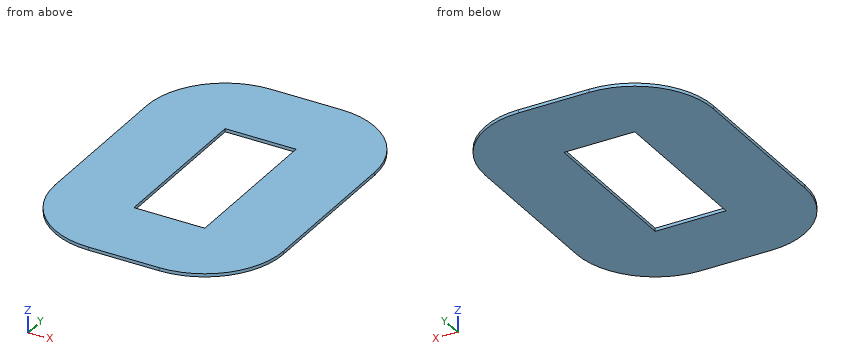
Solid Edge part; units mm, degrees
sketch "Sketch1" plane through (0, 0, 0) normal (0, 0, 1) x (1, 0, 0)
  arc A0 (-55.4402, 24.709) -> (-45.4402, 34.709) centre (-45.4402, 24.709) cw
  line L0 (-36.4402, 34.709) -> (-45.4402, 34.709)
  arc A1 (-36.4402, 34.709) -> (-26.4402, 24.709) centre (-36.4402, 24.709) cw
  line L1 (-26.4402, 4.709) -> (-26.4402, 24.709)
  arc A2 (-26.4402, 4.709) -> (-36.4402, -5.291) centre (-36.4402, 4.709) cw
  line L2 (-45.4402, -5.291) -> (-36.4402, -5.291)
  arc A3 (-45.4402, -5.291) -> (-55.4402, 4.709) centre (-45.4402, 4.709) cw
  line L3 (-55.4402, 24.709) -> (-55.4402, 4.709)
  line L4 (-36.4402, 24.709) -> (-36.4402, 4.709)
  line L5 (-36.4402, 4.709) -> (-45.4402, 4.709)
  line L6 (-45.4402, 4.709) -> (-45.4402, 24.709)
  line L7 (-45.4402, 24.709) -> (-36.4402, 24.709)
extrude "Protrusion1" add sketch "Sketch1" along normal blind 0.4
properties material "Copper"
CAD build for the part. Positions are in the model's coordinates, mm. Coordinates: 2 decimals unless noted, no trailing zeros. Write each loop counter-clockwise with the first axis right and the second up, starting at its lowest first coordinate (ties: lowest second). Pieces come first, ordered by that corner, then holes.
(1) Cut at C-C, the plane z = 0.1. List the corners of the cut face in (x, y), and give its area (3 significant figures).
(2) Cut at D-D, the plane y = 27. List the corners of the cut face in (x, z).
(3) Cut at A-A, the plane y = 6. List the corners of the cut face in (x, z).
(4) Cut at B-B, the plane x = -45. List the corners of the cut face in (y, z).
(5) Drill centre lines: probe 1 along X at (y, z) = (20, 0.1); probe 2 along Y at (x, z) = (-44.5, 0.1); probe 3 along X at (y, z) = (26.5, 0.15). Where is each one in solid material? Low to high.
Geometry says:
1. outline: (-55.44, 4.71) arc R10 ccw to (-45.44, -5.29) - (-36.44, -5.29) arc R10 ccw to (-26.44, 4.71) - (-26.44, 24.71) arc R10 ccw to (-36.44, 34.71) - (-45.44, 34.71) arc R10 ccw to (-55.44, 24.71) - close; hole (-45.44, 4.71) - (-36.44, 4.71) - (-36.44, 24.71) - (-45.44, 24.71) - close
1. area: 894 mm2
2. outline: (-55.17, 0) - (-26.71, 0) - (-26.71, 0.4) - (-55.17, 0.4) - close
3. outline: (-55.44, 0) - (-45.44, 0) - (-45.44, 0.4) - (-55.44, 0.4) - close; (-36.44, 0) - (-26.44, 0) - (-26.44, 0.4) - (-36.44, 0.4) - close
4. outline: (-5.29, 0) - (4.71, 0) - (4.71, 0.4) - (-5.29, 0.4) - close; (24.71, 0) - (34.71, 0) - (34.71, 0.4) - (24.71, 0.4) - close
5. probe 1: x = -55.44 to -45.44, -36.44 to -26.44
5. probe 2: y = -5.29 to 4.71, 24.71 to 34.71
5. probe 3: x = -55.28 to -26.6
